Check sheet for the drawn part. Datum: minimum x, y, z corner. Units: mm. A direction names the side the tool comes from. Give positions to 0.01 mm unless a question says otherwise; leave off trailing zeros. Write each loop counter-clockwise with the first axis right and the second up, starting at its lowest first coordinate (ties: lowest second). Pieces come first, ordered by that corner, then holes.
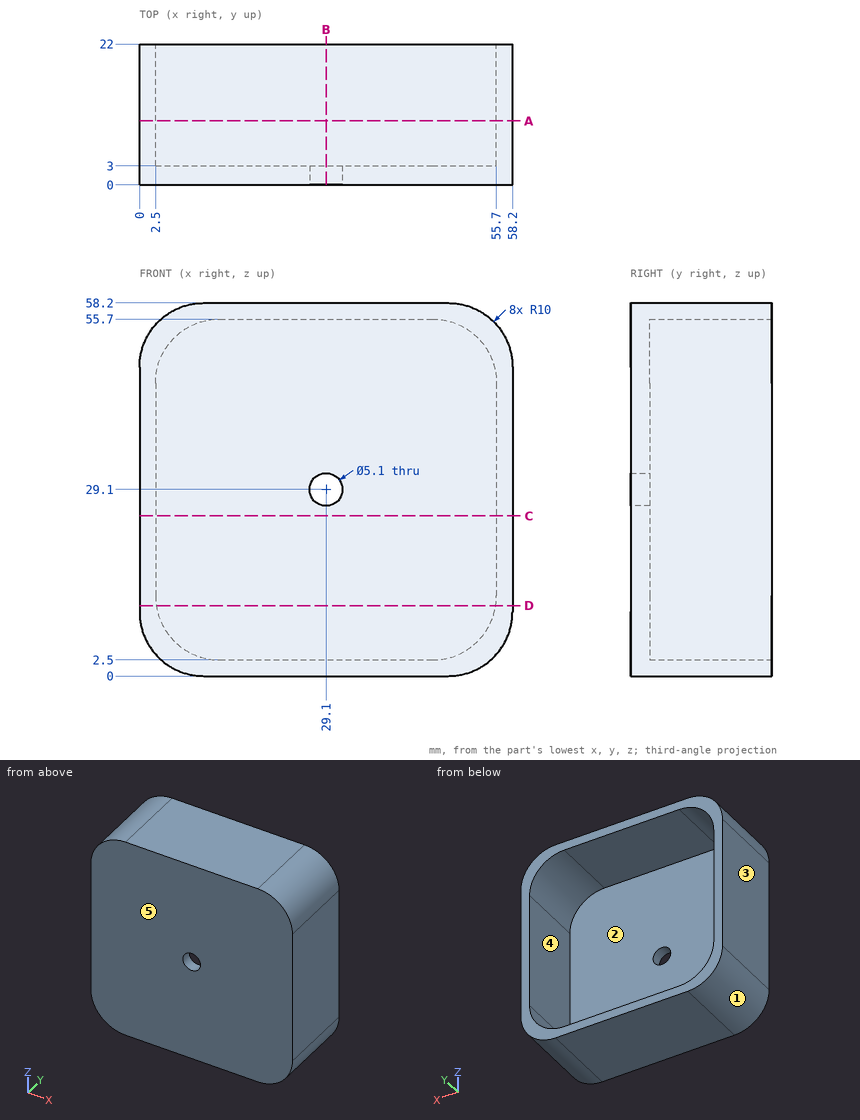
1) Sectioned sample at D-D on z = 11. Record the boundary of the cut face in (x, y), then the cut area to 3 significant figures.
2) Sectioned sample at C-C on z = 25. Record the boundary of the cut face in (x, y).
3) Sectioned sample at A-A on y = 10. Record the boundary of the cut face in (x, z).
4) Access from +Z, -Z, +X, -X, +Y, -Y to the whole of each face (thin tool, end or side, straight path). Record for the marked faces 1 and 2.
5) Gauge pin test, flat end, axial feed: pin 1 (5 mm diameter, centred on x = 14, z = 24, fed in from +Y). Record the tip position at first contact, or that the pin passes through.
6) Sectioned sample at B-B on x = 29.1. Record the boundary of the cut face in (y, z), then the cut area to 3 significant figures.
7) Draft check along X on the marked faces 3, 4 and 5. Enter one of: +X half, -X half, draft (parallel to the pull), parting line (faces both ways), or undercut.
8) Scan lines: L1, parallel to X at y = 1.5, z = 29.1; L2, parallel to X at y = 8.25, z = 25. Record each from-to range of solid material in increasing order.
Answers below:
1. outline: (0, 0) - (58.2, 0) - (58.2, 22) - (55.59, 22) - (55.59, 3) - (2.61, 3) - (2.61, 22) - (0, 22) - close
1. area: 274 mm2
2. outline: (0, 0) - (58.2, 0) - (58.2, 22) - (55.7, 22) - (55.7, 3) - (2.5, 3) - (2.5, 22) - (0, 22) - close
3. outline: (0, 10) arc R10 ccw to (10, 0) - (48.2, 0) arc R10 ccw to (58.2, 10) - (58.2, 48.2) arc R10 ccw to (48.2, 58.2) - (10, 58.2) arc R10 ccw to (0, 48.2) - close; hole (2.5, 12.5) arc R10 ccw to (12.5, 2.5) - (45.7, 2.5) arc R10 ccw to (55.7, 12.5) - (55.7, 45.7) arc R10 ccw to (45.7, 55.7) - (12.5, 55.7) arc R10 ccw to (2.5, 45.7) - close
4. face 1: -Z, -X, +Y, -Y
4. face 2: +Y
5. pin 1: stops at y = 3
6. outline: (0, 0) - (22, 0) - (22, 2.5) - (3, 2.5) - (3, 26.55) - (0, 26.55) - close; (0, 31.65) - (3, 31.65) - (3, 55.7) - (22, 55.7) - (22, 58.2) - (0, 58.2) - close
6. area: 254 mm2
7. face 3: -X half
7. face 4: undercut
7. face 5: draft
8. L1: x = 0 to 26.55, 31.65 to 58.2
8. L2: x = 0 to 2.5, 55.7 to 58.2
